Input: part model. Units: mm. Frame: model coordinates. Face numbers are marked on the shaded views. A direction names the side the tool comes from. Round coordinates to 2 decimals unless told otherwise and drop trailing zeros. Order: outer loops, then holes, each group sorted by start corner. A loop starts at its lowest first (then second) coordinate and runs counter-clockwise, first axis right, second up. Notation, with made-up numbers: (89.5, 54.25) -> (121.5, 54.25) arc R26 cw to (121.5, 89.25) -> close; hole circle Ø10 at (11.5, 16). An arc over 180 degrees is marked (long way). Use a Markdown table: item, result.
from build123d import *

# Parameters (mm, degrees)
F0_R     = 34.3734140818
F1_DEPTH = 44.2854
F2_R     = 34.5672113186
F3_DEPTH = 14.14017
F6_DEPTH = 12.7
F8_DEPTH = 12.7


# Not quite as in the source:
# - a fillet or chamfer that OpenCascade refuses, or shapes differently, is made with other operations: its cross-section is extruded or revolved along the edge and cut away or added


with BuildPart() as f1:
    # F0 (on Front) → F1 (new body)
    with BuildSketch(Plane.XZ):
        Circle(F0_R)
    extrude(amount=F1_DEPTH)

    # F2 (on face) → F3 (join)
    with BuildSketch(Plane.XZ.offset(44.2854)):
        Circle(F2_R)
    extrude(amount=F3_DEPTH)

    # F4: fillet of radius 14.2211905527 on 1 edges, made by hand

    # F4_s1 → F4_t2 (revolve, cut)
    with BuildSketch(Plane.XY):
        with BuildLine():
            ThreePointArc((34.5672113186, -44.2043794473), (30.4019210422, -54.2602797237), (20.3460207659, -58.42557))
            Line((20.3460207659, -58.42557), (34.5672113186, -58.42557))
            Line((34.5672113186, -58.42557), (34.5672113186, -44.2043794473))
        make_face()
    revolve(axis=Axis((0, -58.42557, 0), (0, -1, 0)), mode=Mode.SUBTRACT)

    # F5 (on Top) → F6 (join, symmetric)
    with BuildSketch(Plane.XY):
        Polygon((34.6197038889, -24.2337957025), (34.1581068933, -44.0824255347), (64.1618520021, -44.0824255347), align=None)
    extrude(amount=F6_DEPTH, both=True)

    # F7 (on Top) → F8 (join, symmetric)
    with BuildSketch(Plane.XY):
        Polygon((-55.8531209826, -38.0816757679), (-34.6197001636, -44.544018805), (-33.6965061724, -35.7736945152), (-44.7748154402, -30.6961387396), (-44.7748154402, -17.3098519444), (-34.158103168, -12.6938922331), (-34.158103168, 0), (-55.8531209826, -13.6170834303), align=None)
    extrude(amount=F8_DEPTH, both=True)


solid = f1.part
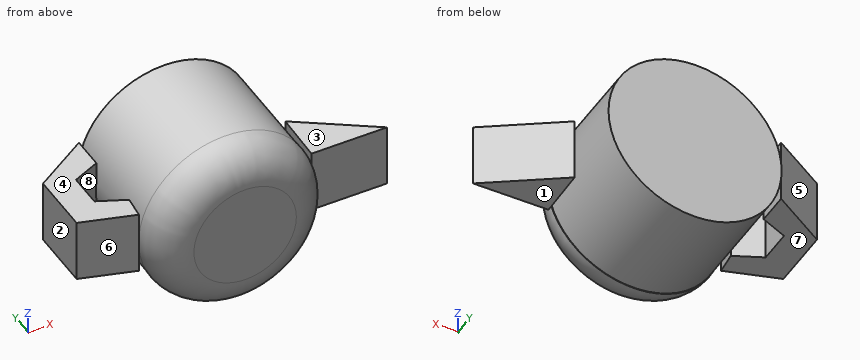
1) Set-up query: the marked faces 1, 2, 3, 4 and 5. Return all of +Z, -Z, +X, -X, +Y, -Y with unobstructed straight access to the full face (end or side cutting, diameter ignored); none if empty.
Answer key:
| item | result |
|---|---|
| face 1 | -Z, +X, +Y, -Y |
| face 2 | +Z, -Z, -X, +Y, -Y |
| face 3 | +Z, +X, +Y, -Y |
| face 4 | +Z, -X, +Y, -Y |
| face 5 | +Z, -Z, -X, +Y |
2) Cut plane D-D on y = -52.5. Return loops of the section in (x, z), and give its area (3 significant figures).
Answer key:
| item | result |
|---|---|
| outline | circle Ø63.79 at (0, 0) |
| area | 3,200 mm^2 |
3) Cut plane A-A on x = 0. Return loops of the section in (y, z), and give its area (3 significant figures).
Answer key:
| item | result |
|---|---|
| outline | (-58.43, -20.35) arc R14.22 ccw to (-44.29, -34.57) -> (-44.29, -34.37) -> (0, -34.37) -> (0, 34.37) -> (-44.29, 34.37) -> (-44.29, 34.57) arc R14.22 ccw to (-58.43, 20.35) -> close |
| area | 3,940 mm^2 |
4) Cut plane C-C on y = -8.5. Return loops of the section in (x, z).
Answer key:
| item | result |
|---|---|
| outline | (-47.7, -12.7) -> (-34.16, -12.7) -> (-34.16, -3.84) arc R34.37 ccw (long way) to (-34.16, 3.84) -> (-34.16, 12.7) -> (-47.7, 12.7) -> close |
5) Ray query, probe 1 along X at (y, z) = (-27.5, 6.5); probe 2 along X at (y, z) = (-28, 8.5); probe 3 along X at (y, z) = (-17, 2.5). Return the intervals inside material, ascending.
Answer key:
| item | result |
|---|---|
| probe 1 | x = -55.85 to -44.77, -33.75 to 33.75, 34.54 to 39.48 |
| probe 2 | x = -55.85 to -44.77, -33.31 to 33.31, 34.53 to 40.23 |
| probe 3 | x = -55.85 to -44.06, -34.28 to 34.28 |
6) Contact query for flat-ended pins moving along their axis: P1, Ø3, axis at y = -37, z = -24, coming from the +X side; P2, Ø7, axis at y = -3, z = 9.5, coming from the +X side; P3, Ø7.5, axis at x = 42, z = -3, coming from the -Y side. Output: stop coordinate, or through.
Answer key:
| item | result |
|---|---|
| P1 | stops at x = 25.99 |
| P2 | stops at x = 33.85 |
| P3 | stops at y = -44.08 |
7) Cut plane B-B on z = 0. Return loops of the section in (x, y), and give its area (3 significant figures).
Answer key:
| item | result |
|---|---|
| outline | (-55.85, -38.08) -> (-34.62, -44.54) -> (-34.37, -42.2) -> (-34.37, -44.29) -> (-34.57, -44.29) arc R14.22 ccw to (-20.35, -58.43) -> (20.35, -58.43) arc R14.22 ccw to (34.57, -44.29) -> (34.37, -44.29) -> (34.37, -44.08) -> (64.16, -44.08) -> (34.62, -24.23) -> (34.37, -34.82) -> (34.37, 0) -> (-34.37, 0) -> (-34.37, -0.14) -> (-55.85, -13.62) -> close; hole (-44.77, -30.7) -> (-34.37, -35.46) -> (-34.37, -12.79) -> (-44.77, -17.31) -> close |
| area | 4,780 mm^2 |
8) Draft query along Y for the marked faces 6, 7 and 8. Return one class per face: released by +Y, released by -Y, zero draft, split by the parting line, or undercut.
Answer key:
| item | result |
|---|---|
| face 6 | released by -Y |
| face 7 | zero draft |
| face 8 | undercut |
